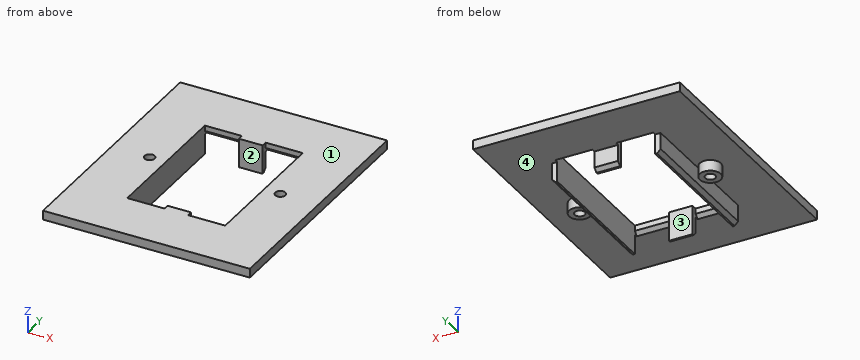
Autodesk Fusion 360 part; units mm, degrees
sketch "Sketch1" plane through (0, 0, 0) normal (0, 0, 1) x (1, 0, 0)
  line L0 (-13.5, 19.5) -> (13.5, 19.5)
  line L1 (13.5, 19.5) -> (13.5, -19.5)
  line L2 (13.5, -19.5) -> (-13.5, -19.5)
  line L3 (-13.5, -19.5) -> (-13.5, 19.5)
  line L4 (-13.5, 19.5) -> (13.5, -19.5) construction
  line L5 (13.5, 19.5) -> (-13.5, -19.5) construction
  line L6 (0, 0) -> (-18, 0) construction
  circle A0 centre (-18, 0) radius 1.4
  circle A1 centre (-18, 0) radius 2.9
  line L7 (0, 50.0244) -> (0, -49.9756) construction
  circle A2 centre (18, 0) radius 2.9
  circle A3 centre (18, 0) radius 1.4
  line L8 (28.5, 34.5) -> (28.5, -34.5)
  line L9 (28.5, -34.5) -> (-28.5, -34.5)
  line L10 (-28.5, -34.5) -> (-28.5, 34.5)
  line L11 (-28.5, 34.5) -> (28.5, 34.5)
  line L12 (-13.5, 19.5) -> (-15, 19.5)
  line L13 (-15, 19.5) -> (-15, -19.5)
  line L14 (-15, -19.5) -> (-13.5, -19.5)
  line L15 (-13.5, -19.5) -> (-13.5, 19.5)
  line L16 (15, -19.5) -> (13.5, -19.5)
  line L17 (15, 19.5) -> (15, -19.5)
  line L18 (13.5, 19.5) -> (15, 19.5)
  line L19 (3.25, 19.5) -> (-3.25, 19.5)
  line L20 (-3.25, 19.5) -> (-3.25, 18)
  line L21 (-3.25, 18) -> (3.25, 18)
  line L22 (3.25, 18) -> (3.25, 19.5)
  line L23 (3.25, 19.5) -> (-3.25, 18) construction
  line L24 (-3.25, 19.5) -> (3.25, 18) construction
  line L25 (-3.25, -19.5) -> (-3.25, -18)
  line L26 (3.25, -18) -> (3.25, -19.5)
  line L27 (-3.25, -18) -> (3.25, -18)
  point P0 (0, 18.75)
  dimension "d2" = 27
  dimension "d3" = 39
  dimension "d4" = -15
  dimension "d5" = 18
  dimension "d6" = 2.8
  dimension "d7" = 1.5
  dimension "d14" = 1.5
  dimension "d19" = 6.5
  dimension "d20" = 1.5
extrude "Extrude1" add sketch "Sketch1" against normal blind 2.5 contours L3 L12 L13 L14 L15 | L1 L16 L17 L18 | A1 | A2 | L8 L9 L10 L11
extrude "Extrude2" add sketch "Sketch1" against normal blind 3 from surface at -2.5 contours A1 | A2
extrude "Extrude3" add sketch "Sketch1" against normal blind 8 contours L3 L12 L13 L14 L15 | L0 L19 L20 L21 L22 | L2 L25 L26 L27 | L1 L16 L17 L18
chamfer "Chamfer2" distance 1 angle 45 2 edges at (15, 0, -8) (-15, 0, -8)
chamfer "Chamfer2" distance 1 angle 45 4 edges at (-8.375, 19.5, -2.5) (8.375, 19.5, -2.5) (8.375, -19.5, -2.5) (-8.375, -19.5, -2.5)
chamfer "Chamfer2" distance 1 angle 45 2 edges at (0, 19.5, -8) (0, -19.5, -8)
equation "d3 = 41 mm - 2 mm"
equation "d5 = ( 36 / 2 ) * 1 mm"
Model file for the job. Use its own axes, mm. Face numbers are marked on the shaded views. A direction names the side the tool comes from. Give positions to 0.01 mm unless a question says otherwise; leave off trailing zeros. Loops run counter-clockwise (first coordinate to the right, second up) from the corner with the lowest first, then second, coordinate; pieces in that order, holes last. Notation, with made-up numbers: (-19.75, 46) - (22.25, 46) arc R20 ccw to (22.25, 74) - close; hole circle Ø8 at (7, 67). An arc over 180 degrees is marked (long way). Use one line per item in the form item = value.
(1) 3-axis set-ups, long thin cutter, end or side, ignore diameter. For the marked faces 1 and 2: which of +Z, -Z, +X, -X, +Y, -Y reach the whole face in a straight line?
Determined:
face_1 = +Z, +X, -X, +Y, -Y
face_2 = +Z, -Z
(2) Cut at A-A (z = -4.25). Give the cut face in (x, y), then the cut area to 3 significant figures.
Determined:
outline = circle Ø5.8 at (-18, 0); (-15, -19.5) - (-13.5, -19.5) - (-13.5, 19.5) - (-15, 19.5) - close; (-3.25, -19.5) - (3.25, -19.5) - (3.25, -18) - (-3.25, -18) - close; (-3.25, 18) - (3.25, 18) - (3.25, 19.5) - (-3.25, 19.5) - close; (13.5, -19.5) - (15, -19.5) - (15, 19.5) - (13.5, 19.5) - close; circle Ø5.8 at (18, 0); hole circle Ø2.8 at (-18, 0); hole circle Ø2.8 at (18, 0)
area = 177 mm^2
(3) Drop flat-ended pins along their axis: P1, Ø3.5, axis at x = -1.5, z = -4.5, coming from the -Y side; P2, Ø1.2, axis at x = 14.5, z = -6, coming from the +Y side; P3, Ø1.3, axis at y = 1.5, z = -3.5, coming from the -X side. Give the stop position or say it passes through.
Determined:
P1 = -19.5
P2 = 19.5
P3 = -20.77
(4) Pull direction Y, two halves, no side cores. Call the marked faces 3 and 4: pulls with the +Y half, pulls with the -Y half, needs draft (parallel to the pull), parting line crosses it, or undercut.
Determined:
face_3 = undercut
face_4 = needs draft
(5) Cut at D-D (z = -0.75). Give the cut face in (x, y), then the cut area to 3 significant figures.
Determined:
outline = (-28.5, -34.5) - (28.5, -34.5) - (28.5, 34.5) - (-28.5, 34.5) - close; hole circle Ø2.8 at (-18, 0); hole (-13.5, -19.5) - (-3.25, -19.5) - (-3.25, -18) - (3.25, -18) - (3.25, -19.5) - (13.5, -19.5) - (13.5, 19.5) - (3.25, 19.5) - (3.25, 18) - (-3.25, 18) - (-3.25, 19.5) - (-13.5, 19.5) - close; hole circle Ø2.8 at (18, 0)
area = 2,890 mm^2
(6) Cut at C-C (y = 12). Give the cut face in (x, z).
Determined:
outline = (-28.5, -2.5) - (-15, -2.5) - (-15, -7) - (-14, -8) - (-13.5, -8) - (-13.5, 0) - (-28.5, 0) - close; (13.5, -8) - (14, -8) - (15, -7) - (15, -2.5) - (28.5, -2.5) - (28.5, 0) - (13.5, 0) - close
(7) Drill centre lines: L1, parallel to Y at x = -18, z = -1.75; L2, parallel to X at y = -19, z = -6.5; L3, parallel to X at y = -15, z = -3.75. Where is each one in solid material? Low to high.
Determined:
L1 = -34.5 to -1.4, 1.4 to 34.5
L2 = -15 to -13.5, -3.25 to 3.25, 13.5 to 15
L3 = -15 to -13.5, 13.5 to 15
(8) Cut at B-B (x = -10). Give the cut face in (y, z).
Determined:
outline = (-34.5, -2.5) - (-20.5, -2.5) - (-19.5, -1.5) - (-19.5, 0) - (-34.5, 0) - close; (19.5, -1.5) - (20.5, -2.5) - (34.5, -2.5) - (34.5, 0) - (19.5, 0) - close
